Source: CAD feature listing. Evaluate the final solid. Frame: model axes, mm. Face numbers are marked on the shaded views. Coordinates: 2 decimals unless noted, no trailing zeros. Order: outer loops, then holes, each group sorted by start corner. A loop starts at its lowest first (then second) coordinate and runs counter-clockwise, first axis right, second up. Notation, with made-up numbers: (45, 23) -> (61, 23) arc R16 ccw to (61, 33) -> close; hole circle Ø2 at (-10, 64.25). An arc over 180 degrees is marked (long way). Put each result on its own line as item: value.
from build123d import *

# Parameters (mm, degrees)
EXTRUDE_2_DEPTH      = 8
EXTRUDE_2_DEPTH_BACK = 3
SKETCH_3_W           = 294.4
SKETCH_3_H           = 157.879
SKETCH_2_W           = 290.4
SKETCH_2_H           = 149.879
CUT_EXTRUDE_2_DEPTH  = 3
SKETCH_5_R           = 8.15
CUT_EXTRUDE_3_DEPTH  = 7


with BuildPart() as part:
    # 草图3 → 凸台-拉伸2 (new, two sides: drawn at the far end of the back side and taken through both)
    with BuildSketch(Plane.XY.offset(-EXTRUDE_2_DEPTH_BACK)):
        with Locations((103.122, -9.5885)):
            Rectangle(SKETCH_3_W, SKETCH_3_H)
    extrude(amount=EXTRUDE_2_DEPTH + EXTRUDE_2_DEPTH_BACK)

    # 草图2 → 切除-拉伸2 (cut)
    with BuildSketch(Plane.XY):
        with Locations((105.122, -9.5885)):
            Rectangle(SKETCH_2_W, SKETCH_2_H)
    extrude(amount=-CUT_EXTRUDE_2_DEPTH, mode=Mode.SUBTRACT)

    # 草图5 → 切除-拉伸3 (cut)
    with BuildSketch(Plane.XY):
        with Locations((-28.645, 19.55)):
            Circle(SKETCH_5_R)
        with Locations((-9.52, 19.55)):
            Circle(SKETCH_5_R)
        with Locations((9.53, 19.55)):
            Circle(SKETCH_5_R)
        with Locations((28.58, 19.55)):
            Circle(SKETCH_5_R)
        with Locations((47.63, 19.55)):
            Circle(SKETCH_5_R)
        with Locations((66.68, 19.55)):
            Circle(SKETCH_5_R)
        with Locations((85.73, 19.55)):
            Circle(SKETCH_5_R)
        with Locations((104.78, 19.55)):
            Circle(SKETCH_5_R)
        with Locations((123.83, 19.55)):
            Circle(SKETCH_5_R)
        with Locations((142.88, 19.55)):
            Circle(SKETCH_5_R)
        with Locations((161.93, 19.55)):
            Circle(SKETCH_5_R)
        with Locations((180.98, 19.55)):
            Circle(SKETCH_5_R)
        with Locations((228.66, 19.55)):
            Circle(SKETCH_5_R)
        with Locations((171.45, 0)):
            Circle(SKETCH_5_R)
        with Locations((152.4, 0)):
            Circle(SKETCH_5_R)
        with Locations((133.35, 0)):
            Circle(SKETCH_5_R)
        with Locations((114.3, 0)):
            Circle(SKETCH_5_R)
        with Locations((95.25, 0)):
            Circle(SKETCH_5_R)
        with Locations((76.2, 0)):
            Circle(SKETCH_5_R)
        with Locations((57.15, 0)):
            Circle(SKETCH_5_R)
        with Locations((38.1, 0)):
            Circle(SKETCH_5_R)
        with Locations((19.05, 0)):
            Circle(SKETCH_5_R)
        Circle(SKETCH_5_R)
        with Locations((-21.495, -19.05)):
            Circle(SKETCH_5_R)
        with Locations((4.76, -19.05)):
            Circle(SKETCH_5_R)
        with Locations((23.81, -19.05)):
            Circle(SKETCH_5_R)
        with Locations((42.86, -19.05)):
            Circle(SKETCH_5_R)
        with Locations((61.91, -19.05)):
            Circle(SKETCH_5_R)
        with Locations((80.96, -19.05)):
            Circle(SKETCH_5_R)
        with Locations((100.01, -19.05)):
            Circle(SKETCH_5_R)
        with Locations((119.06, -19.05)):
            Circle(SKETCH_5_R)
        with Locations((138.11, -19.05)):
            Circle(SKETCH_5_R)
        with Locations((157.16, -19.05)):
            Circle(SKETCH_5_R)
        with Locations((176.21, -19.05)):
            Circle(SKETCH_5_R)
        with Locations((195.26, -19.05)):
            Circle(SKETCH_5_R)
        with Locations((226.28, -19.05)):
            Circle(SKETCH_5_R)
        with Locations((185.74, -38.1)):
            Circle(SKETCH_5_R)
        with Locations((166.69, -38.1)):
            Circle(SKETCH_5_R)
        with Locations((147.64, -38.1)):
            Circle(SKETCH_5_R)
        with Locations((128.59, -38.1)):
            Circle(SKETCH_5_R)
        with Locations((109.54, -38.1)):
            Circle(SKETCH_5_R)
        with Locations((90.49, -38.1)):
            Circle(SKETCH_5_R)
        with Locations((71.44, -38.1)):
            Circle(SKETCH_5_R)
        with Locations((52.39, -38.1)):
            Circle(SKETCH_5_R)
        with Locations((33.34, -38.1)):
            Circle(SKETCH_5_R)
        with Locations((14.29, -38.1)):
            Circle(SKETCH_5_R)
        with Locations((-16.73, -38.1)):
            Circle(SKETCH_5_R)
        with Locations((-27.455, -57.53)):
            Circle(SKETCH_5_R)
        with Locations((-2.38, -57.53)):
            Circle(SKETCH_5_R)
        with Locations((21.43, -57.53)):
            Circle(SKETCH_5_R)
        with Locations((92.87, -57.53)):
            Circle(SKETCH_5_R)
    extrude(amount=CUT_EXTRUDE_3_DEPTH, mode=Mode.SUBTRACT)


solid = part.part
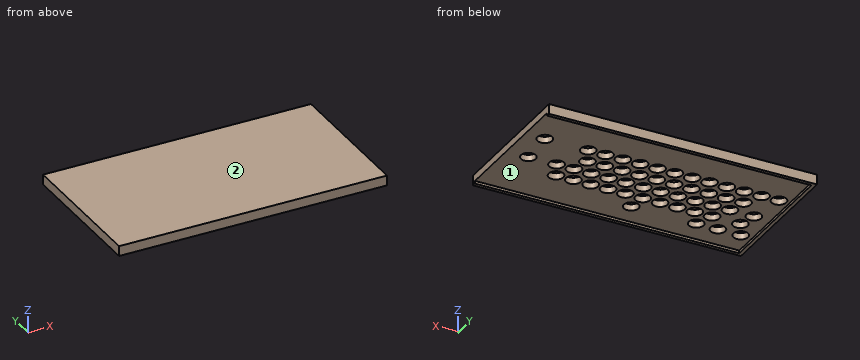
1. Pull-direction query (Y, two-part tool) for the marked faces 1 and 2; classes: pulls with the +Y half, pulls with the -Y half, needs draft (parallel to the pull), parting line crosses it, or undercut.
Numbers:
face 1: undercut
face 2: needs draft
2. First-contact query: pin 1 (13 mm diameter, centred on x = 126, y = 17, fed in from -Z); pin 2 (8 mm diameter, centred on x = 3.5, y = -22.5, fed in from -Z). Flat tips, straight axial feed; report the tip coordinate or a pass-through.
Numbers:
pin 1: stops at z = 0
pin 2: stops at z = 7
3. Cut plane A-A on y = 32. Output: boundary loops of the cut face in (x, z).
Numbers:
outline: (-44.08, -3) -> (-40.08, -3) -> (-40.08, 0) -> (250.32, 0) -> (250.32, 8) -> (-44.08, 8) -> close
4. Ray query, line 1 along Y through (x, z) = (-17, -1.75); line 2 along Y through (x, z) = (126, 3); line 3 along Y through (x, z) = (66.5, 4.75). Return the intervals inside material, ascending.
Numbers:
line 1: y = -88.53 to -84.53, 65.35 to 69.35
line 2: y = -88.53 to -45.83, -30.37 to -23.32, -14.78 to -3.52, 3.52 to 11.69, 27.41 to 69.35
line 3: y = -88.53 to -44.58, -31.62 to -25.78, -12.32 to 11.4, 27.7 to 69.35
